from build123d import *

# Parameters (mm, degrees)
F0_W     = 42
F0_H     = 42
F1_DEPTH = 33
F2_R     = 11
F3_DEPTH = 2
F4_R     = 2.5
F5_DEPTH = 10
F6_R     = 1.5
F7_DEPTH = 33.001
F8_SIZE  = 3


with BuildPart() as f1:
    # F0 (on Top) → F1 (new body)
    with BuildSketch(Plane.XY):
        Rectangle(F0_W, F0_H)
    extrude(amount=F1_DEPTH)

    # F2 (on face) → F3 (join)
    with BuildSketch(Plane.XY.offset(33)):
        Circle(F2_R)
    extrude(amount=F3_DEPTH)

    # F4 (on face) → F5 (join)
    with BuildSketch(Plane.XY.offset(35)):
        Circle(F4_R)
    extrude(amount=F5_DEPTH)

    # F6 (on face) → F7 (cut, through all)
    with BuildSketch(Plane.XY.offset(33)):
        with Locations((-15.5, 15.5)):
            Circle(F6_R)
        with Locations((15.5, 15.5)):
            Circle(F6_R)
        with Locations((15.5, -15.5)):
            Circle(F6_R)
        with Locations((-15.5, -15.5)):
            Circle(F6_R)
    extrude(amount=-F7_DEPTH, mode=Mode.SUBTRACT)

    # F8
    f8_edges = [f1.edges().sort_by_distance(p)[0] for p in [
        (-21, 21, 16.5),
        (21, 21, 16.5),
        (21, -21, 16.5),
        (-21, -21, 16.5),
    ]]
    chamfer(f8_edges, length=F8_SIZE)


solid = f1.part
Geometry check sheet. Reference: the model listing, model coordinates, mm. A direction names the side the tool comes from. Give positions to 0.01 mm unless a question says otherwise; leave off trailing zeros. Loops run counter-clockwise (first coordinate to the right, second up) from the corner with the lowest first, then second, coordinate; pieces in that order, holes last. Notation, with made-up numbers: (81, 1) -> (108, 1) arc R14 ccw to (108, 21) -> close; hole circle Ø2 at (65, 65). An arc over 180 degrees is marked (long way). Answer in a Markdown table with one row per item. Add a question column.
1) Draft check along X on faces 3 (the face through (-19, -20, 16)), 4 (the face through (14, 15.57, 16.73)), 5 (the face through (0, 21, 16)). Enter one of: pulls with the +X half, pulls with the -X half, needs draft (parallel to the pull), parting line crosses it, or undercut.
2) Gauge pin test, flat ends, axial feed: P1, Ø21, axis at x = 1, y = 7.5, coming from the +Z side; P2, Ø2, axis at x = -13.5, y = 6, coming from the +Z side. Record the tip position at first contact, or that the pin passes through.
3) Cross-section at B-B on x = -15.5. Record the boundary of the cut face in (y, z), and give its area (3 significant figures).
4) Cross-section at A-A on z = 19. Record the boundary of the cut face in (x, y).
5) Material ranges on probe 1 along Y at (x, z) = (-15.5, 17.5); probe 2 along X at (y, z) = (-15, 20), recorded low to high. Write a range as from..to.
6) Set-up check for faces 1 (the face through (20, -19, 16)), 2 (the face through (-10, 10, 33)): record each of +Z, -Z, +X, -X, +Y, -Y from which the full face is reachable in a straight line by a thin tool's end or side.
7) Cross-section at D-D on x = 0. Record the boundary of the cut face in (y, z).
Outcome:
| question | item | result |
|---|---|---|
| 1 | face 3 | pulls with the -X half |
| 1 | face 4 | undercut |
| 1 | face 5 | needs draft |
| 2 | P1 | stops at z = 45 |
| 2 | P2 | stops at z = 33 |
| 3 | outline | (-21, 0) -> (-17, 0) -> (-17, 33) -> (-21, 33) -> close; (-14, 0) -> (14, 0) -> (14, 33) -> (-14, 33) -> close; (17, 0) -> (21, 0) -> (21, 33) -> (17, 33) -> close |
| 3 | area | 1,190 mm^2 |
| 4 | outline | (-21, -18) -> (-18, -21) -> (18, -21) -> (21, -18) -> (21, 18) -> (18, 21) -> (-18, 21) -> (-21, 18) -> close; hole circle Ø3 at (-15.5, -15.5); hole circle Ø3 at (-15.5, 15.5); hole circle Ø3 at (15.5, -15.5); hole circle Ø3 at (15.5, 15.5) |
| 5 | probe 1 | y = -21..-17, -14..14, 17..21 |
| 5 | probe 2 | x = -21..-16.91, -14.09..14.09, 16.91..21 |
| 6 | face 1 | +Z, -Z, +X, -Y |
| 6 | face 2 | +Z |
| 7 | outline | (-21, 0) -> (21, 0) -> (21, 33) -> (11, 33) -> (11, 35) -> (2.5, 35) -> (2.5, 45) -> (-2.5, 45) -> (-2.5, 35) -> (-11, 35) -> (-11, 33) -> (-21, 33) -> close |
